Build history of the part. All positions in model axes, mm. A direction names the side the tool comes from. Give positions to 0.01 mm unless a question says otherwise; leave off trailing zeros. Order: outer loops, then holes, each group sorted by start corner. A loop starts at its lowest first (then second) coordinate and runs counter-clockwise, first axis right, second up. Notation, with made-up numbers: (-3.75, 0) -> (30.25, 0) arc R25 ccw to (30.25, 17) -> close; hole circle Ø6 at (38, 71). An arc over 180 degrees is marked (long way). Use a Markdown table: item, result. Add a question column.
```python
from build123d import *

# Parameters (mm, degrees)
F0_W     = 2.5
F0_H     = 20
F1_DEPTH = 3.5
F0_W_2   = 5
F2_DEPTH = 28.5
F3_R     = 2.271243
F4_DEPTH = 5
F5_R     = 2


with BuildPart() as f1:
    # F0 (on Top) → F1 (new body)
    with BuildSketch(Plane.XY):
        with BuildLine():
            Line((15.000003, 19.129753), (-49.999997, 19.129753))
            ThreePointArc((-49.999997, 19.129753), (-53.535531, 17.665286), (-54.999997, 14.129753))
            Line((-54.999997, 14.129753), (-54.999997, 9.129753))
            Line((-54.999997, 9.129753), (-52.499997, 9.129753))
            Line((-52.499997, 9.129753), (-47.499997, 9.129753))
            Line((-47.499997, 9.129753), (-44.999997, 9.129753))
            Line((-44.999997, 9.129753), (-44.999997, -10.870247))
            Line((-44.999997, -10.870247), (-47.499997, -10.870247))
            Line((-47.499997, -10.870247), (-52.499997, -10.870247))
            Line((-52.499997, -10.870247), (-54.999997, -10.870247))
            Line((-54.999997, -10.870247), (-54.999997, -15.870247))
            ThreePointArc((-54.999997, -15.870247), (-53.535531, -19.405781), (-49.999997, -20.870247))
            Line((-49.999997, -20.870247), (15.000003, -20.870247))
            ThreePointArc((15.000003, -20.870247), (18.535537, -19.405781), (20.000003, -15.870247))
            Line((20.000003, -15.870247), (20.000003, 14.129753))
            ThreePointArc((20.000003, 14.129753), (18.535537, 17.665286), (15.000003, 19.129753))
        make_face()
        with Locations((-53.749997, -0.870247)):
            Rectangle(F0_W, F0_H)
        with Locations((-46.249997, -0.870247)):
            Rectangle(F0_W, F0_H)
    extrude(amount=F1_DEPTH)

    # F0 (on Top) → F2 (join)
    with BuildSketch(Plane.XY):
        with Locations((-49.999997, -0.870247)):
            Rectangle(F0_W_2, F0_H)
    extrude(amount=F2_DEPTH)

    # F3 (on face) → F4 (cut)
    with BuildSketch(Plane(origin=(-52.499997, 0, 0), x_dir=(0, -1, 0), z_dir=(-1, 0, 0))):
        with Locations((0.870247, 16.3)):
            Circle(F3_R)
    extrude(amount=-F4_DEPTH, mode=Mode.SUBTRACT)

    # F5
    f5_edges = [f1.edges().sort_by_distance(p)[0] for p in [
        (-52.499997, -0.870247, 28.5),
        (-47.499997, -0.870247, 28.5),
        (-47.499997, -10.870247, 16),
        (-52.499997, -10.870247, 16),
        (-52.499997, 9.129753, 16),
        (-47.499997, 9.129753, 16),
    ]]
    fillet(f5_edges, radius=F5_R)


solid = f1.part
```
(1) Band-saw the part on C-C on z = 5.5. Give the cut face in (x, y), plus the area to 3 significant figures.
(2) Band-saw the part on D-D on y = 13. Give the cut face in (x, z), plus the area to 4 significant figures.
(3) Wall check: probe 1 along X at (y, z) = (0.5, 6.75); probe 2 along Z at (x, y) = (-12, -14.5). Give the ranges that are in metal, low to high.
(4) Band-saw the part on B-B on y = -1. Give the cut face in (x, z).
(5) Pin check, flat tips, straight feed: pin 1 Ø0.5 at (x, z) = (-50, 18) entering from -Y; pin 2 Ø20 at (x, y) = (-8, 7.5) entering from +Z; pin 3 Ø12 at (y, z) = (7, 25.5) entering from -X. Stop position of each tip, or through.
(6) Mould opens along Z. For faces 6 (the face through (-18, -1, 0)), 7 (the face through (-18, -1, 3.5)), 8 (the face through (-50.03, -0.57, 18.55)), 9 (the face through (18.5, -19.44, 1.73)) say: released by +Z, released by -Z, zero draft, split by the parting line, or undercut.
(7) Tool access for faces 1 (the face through (-51.9, -10.3, 16.2)), 2 (the face through (-47.5, -3, 15)), 3 (the face through (-52.5, -3, 15)), 4 (the face through (-48.1, 8.56, 16.18)), 5 (the face through (-48.1, -10.3, 16.2)): list every direction of +Z, -Z, +X, -X, +Y, -Y with a clear straight run to the whole face (end or side of a thin tool).
(8) Band-saw the part on A-A on z = 16.3. Give the cut face in (x, y), plus the area to 3 significant figures.
Response:
| question | item | result |
|---|---|---|
| 1 | outline | (-52.5, -8.87) arc R2 ccw to (-50.5, -10.87) -> (-49.5, -10.87) arc R2 ccw to (-47.5, -8.87) -> (-47.5, 7.13) arc R2 ccw to (-49.5, 9.13) -> (-50.5, 9.13) arc R2 ccw to (-52.5, 7.13) -> close |
| 1 | area | 96.6 mm² |
| 2 | outline | (-55, 0) -> (20, 0) -> (20, 3.5) -> (-55, 3.5) -> close |
| 2 | area | 262.5 mm² |
| 3 | probe 1 | x = -52.5 to -47.5 |
| 3 | probe 2 | z = 0 to 3.5 |
| 4 | outline | (-55, 0) -> (20, 0) -> (20, 3.5) -> (-47.5, 3.5) -> (-47.5, 14.03) -> (-52.5, 14.03) -> (-52.5, 3.5) -> (-55, 3.5) -> close; (-52.5, 18.57) -> (-47.5, 18.57) -> (-47.5, 26.5) arc R2 ccw to (-49.5, 28.5) -> (-50.5, 28.5) arc R2 ccw to (-52.5, 26.5) -> close |
| 5 | pin 1 | stops at y = -10.87 |
| 5 | pin 2 | stops at z = 3.5 |
| 5 | pin 3 | stops at x = -52.5 |
| 6 | face 6 | released by -Z |
| 6 | face 7 | released by +Z |
| 6 | face 8 | undercut |
| 6 | face 9 | zero draft |
| 7 | face 1 | +Z, -X, -Y |
| 7 | face 2 | +Z, +X, +Y, -Y |
| 7 | face 3 | +Z, -X, +Y, -Y |
| 7 | face 4 | +Z, +X, +Y |
| 7 | face 5 | +Z, +X, -Y |
| 8 | outline | (-52.5, -8.87) arc R2 ccw to (-50.5, -10.87) -> (-49.5, -10.87) arc R2 ccw to (-47.5, -8.87) -> (-47.5, -3.14) -> (-52.5, -3.14) -> close; (-52.5, 1.4) -> (-47.5, 1.4) -> (-47.5, 7.13) arc R2 ccw to (-49.5, 9.13) -> (-50.5, 9.13) arc R2 ccw to (-52.5, 7.13) -> close |
| 8 | area | 73.9 mm² |
